The model under review builds one solid part; all positions refer to its coordinate system, in mm. A direction names the side the tool comes from. Coordinates: 2 decimals unless noted, no trailing zeros. Order: outer loops, then holes, each group sorted by start corner. A loop starts at its lowest first (then second) coordinate and runs counter-clockwise, first axis right, second up.
```python
from build123d import *

# Parameters (mm, degrees)
EXTRUDE_1_DEPTH                  = 10.5
SKETCH_2_W                       = 102.00000000000001
SKETCH_2_H                       = 75.00000000000009
EXTRUDE_2_DEPTH                  = 19.4993693487819
EXTRUDE_3_DEPTH                  = 18.000000000000004
SKETCH_4_W                       = 18.000000000000004
SKETCH_4_H                       = 140
EXTRUDE_4_DEPTH                  = 70.0006306512181
EXTRUDE_START                    = 10.499999999999998
EXTRUDE_5_DEPTH                  = 10.499999999999998
CUT_EXTRUDE_1_REACH              = 194.401
SKETCH_7_W                       = 4.000000000000014
SKETCH_7_H                       = 29.999999999999993
CUT_EXTRUDE_2_DEPTH              = 201.0099997500125
CUT_EXTRUDE_3_DEPTH              = 210.76176963403032
CUT_EXTRUDE_4_DEPTH              = 210.76176963403032
EXTRUDE_6_DEPTH                  = 0.7500000000000007
HOLE_WIZARD_M521_D               = 61.5
EXTRUDE_7_DEPTH                  = 5.749999999999998
HOLE_WIZARD_6_7_6_7_1_AT_2_COUNT = 2
HOLE_WIZARD_6_7_6_7_1_AT_2_PITCH = 45
HOLE_WIZARD_4_0_4_1_AT_2_COUNT   = 2
HOLE_WIZARD_4_0_4_1_AT_2_PITCH   = 49.49747468305833
CHAMFER_1_SIZE                   = 0.9999999999999991
EXTRUDE_START_2                  = -16.249369
SKETCH_28_R                      = 3.35
SKETCH_28_R_2                    = 9.999999999999993
SKETCH_28_R_3                    = 3.350000000000003
EXTRUDE_8_DEPTH                  = 16.249369
SKETCH_30_R                      = 3.0000000000000018
CUT_EXTRUDE_5_DEPTH              = 7
EXTRUDE_START_3                  = -21.000000000000007
SKETCH_32_R                      = 2.9999999999999933
EXTRUDE_9_DEPTH                  = 21.000000000000007


with BuildPart() as part:
    # Эскиз1 → Бобышка-Вытянуть1 (new body)
    with BuildSketch(Plane(origin=(29.9993693487819, 0, 0), x_dir=(0, 0, -1), z_dir=(1, 0, 0))):
        with BuildLine():
            Line((14.919229074297327, 90.0005475751909), (0, 90.0005475751909))
            Line((0, 90.0005475751909), (0, 15.0005475751908))
            Line((0, 15.0005475751908), (102.00000000000001, 15.0005475751908))
            Line((102.00000000000001, 15.0005475751908), (85.69382268537409, 20.93551075238141))
            ThreePointArc((85.69382268537409, 20.93551075238141), (74.94644857866616, 27.70982740688085), (67.9664449575318, 38.324768093192546))
            ThreePointArc((67.9664449575318, 38.324768093192546), (24.088528585175357, 46.3477790832992), (14.919229074297327, 90.0005475751909))
        make_face()
    extrude(amount=-EXTRUDE_1_DEPTH)

    # Эскиз2 → Бобышка-Вытянуть2 (add)
    with BuildSketch(Plane.ZY.offset(-19.4993693487819)):
        with Locations((-51.00000000000001, 52.50054757519085)):
            Rectangle(SKETCH_2_W, SKETCH_2_H)
    extrude(amount=EXTRUDE_2_DEPTH)

    # Эскиз3 → Бобышка-Вытянуть3 (add)
    with BuildSketch(Plane.XY):
        Polygon((29.999369348781915, -6.94e-15), (3.47e-15, 15.000547575190799), (0, 124.997494914823), (29.997641385548, 140), (29.999369348781904, 140), align=None)
    extrude(amount=EXTRUDE_3_DEPTH)

    # Эскиз4 → Бобышка-Вытянуть4 (add)
    with BuildSketch(Plane(origin=(29.9993693487819, 0, 0), x_dir=(0, 0, -1), z_dir=(1, 0, 0))):
        with Locations((-9.000000000000002, 70)):
            Rectangle(SKETCH_4_W, SKETCH_4_H)
    extrude(amount=EXTRUDE_4_DEPTH)

    # Эскиз5 → Бобышка-Вытянуть5 (add)
    with BuildSketch(Plane(origin=(19.4993693487819, 0, 0), x_dir=(0, 0, -1), z_dir=(1, 0, 0)).offset(EXTRUDE_START)):
        with BuildLine():
            Line((89.08077092570272, 90.0005475751909), (102.00000000000001, 90.0005475751909))
            Line((102.00000000000001, 90.0005475751909), (102.00000000000001, 23.000547575190808))
            Line((102.00000000000001, 23.000547575190808), (91.92678266011816, 26.666898850201964))
            ThreePointArc((91.92678266011816, 26.666898850201964), (81.8910585435448, 32.765618882150974), (74.9654117449494, 42.24958224106233))
            ThreePointArc((74.9654117449494, 42.24958224106233), (90.35915387380979, 63.660894475956894), (89.08077092570272, 90.0005475751909))
        make_face()
    extrude(amount=-EXTRUDE_5_DEPTH)

    # Эскиз6 → Вырез-Вытянуть1 (cut, up to next)
    with BuildSketch(Plane(origin=(16.2493693487819, 0, 0), x_dir=(0, -1, 0), z_dir=(-1, 0, 0)), mode=Mode.PRIVATE) as cut_extrude_1_sk1:
        with BuildLine():
            Line((-90.0005475751909, -14.919229074297327), (-90.0005475751909, -89.08077092570272))
            ThreePointArc((-90.0005475751909, -89.08077092570272), (-34.999999999999936, -52), (-90.0005475751909, -14.919229074297327))
        make_face()
    cut_extrude_1_tool1 = extrude(cut_extrude_1_sk1.sketch, amount=-CUT_EXTRUDE_1_REACH, mode=Mode.PRIVATE) & part.part
    add(cut_extrude_1_tool1.solids().sort_by_distance((16.249369, 65.774947, -52))[0], mode=Mode.SUBTRACT)

    # Эскиз7 → Вырез-Вытянуть2 (cut, through all)
    with BuildSketch(Plane.ZY):
        with Locations((-100, 75.0005475751909)):
            Rectangle(SKETCH_7_W, SKETCH_7_H)
    extrude(amount=-CUT_EXTRUDE_2_DEPTH, mode=Mode.SUBTRACT)

    # Эскиз8 → Вырез-Вытянуть3 (cut, through all)
    with BuildSketch(Plane.XY.offset(18.000000000000004)):
        with BuildLine():
            Line((64, 140), (45.999999999999986, 140))
            Line((45.999999999999986, 140), (46, 120))
            ThreePointArc((46, 120), (55, 111), (64, 120))
            Line((64, 120), (64, 140))
        make_face()
    extrude(amount=-CUT_EXTRUDE_3_DEPTH, mode=Mode.SUBTRACT)

    # Эскиз9 → Вырез-Вытянуть4 (cut, through all)
    with BuildSketch(Plane.XY.offset(18.000000000000004)):
        with BuildLine():
            Line((46.00000000000001, 0), (64, 0))
            Line((64, 0), (64, 20.000000000000004))
            ThreePointArc((64, 20.000000000000004), (55, 29), (45.999999999999986, 20.000000000000004))
            Line((45.999999999999986, 20.000000000000004), (46.00000000000001, 0))
        make_face()
    extrude(amount=-CUT_EXTRUDE_4_DEPTH, mode=Mode.SUBTRACT)

    # Эскиз10 → Бобышка-Вытянуть6 (add)
    with BuildSketch(Plane(origin=(16.2493693487819, 0, 0), x_dir=(0, 0, -1), z_dir=(1, 0, 0))):
        with BuildLine():
            Line((15.729542704227807, 90.0005475751909), (88.27045729577222, 90.00054757519085))
            ThreePointArc((88.27045729577222, 90.00054757519085), (51.999999999999986, 35.75000000000001), (15.729542704227807, 90.0005475751909))
        make_face()
    extrude(amount=EXTRUDE_6_DEPTH)

    # Отверстие с зазором M521 (through all)
    with Locations(Plane(origin=(16.999369348781904, 0, 0), x_dir=(0, 0, -1), z_dir=(1, 0, 0))):
        with Locations((52, 75)):
            Hole(HOLE_WIZARD_M521_D / 2)

    # Эскиз20 → Диаметр отверстия Ø4.0 (4)1 (revolve, cut)
    with BuildSketch(Plane(origin=(16.999369348781904, 75, -17), x_dir=(0, 0, -1), z_dir=(0, 1, 0))):
        Polygon((0, 0), (-4.16e-15, 16.999369348781904), (1.9999999999999978, 16.999369348781904), (1.9999999999999896, -1.31e-15), align=None)
    hole_wizard_4_0_4_1 = revolve(axis=Axis((23.349369348781895, 75, -17), (-1, 0, 0)), mode=Mode.SUBTRACT)

    # Диаметр отверстия Ø4.0 (4)1 at 2: Диаметр отверстия Ø4.0 (4)1 ×2
    with Locations(*[Vector(0, -0.7071067811865475, -0.7071067811865477) * (i * HOLE_WIZARD_4_0_4_1_AT_2_PITCH) for i in range(1, HOLE_WIZARD_4_0_4_1_AT_2_COUNT)]):
        add(hole_wizard_4_0_4_1, mode=Mode.SUBTRACT)

    # Эскиз22 → Диаметр отверстия Ø6.0 (6)1 (revolve, cut)
    with BuildSketch(Plane(origin=(29.9993693487819, 40.0005475751908, -90), x_dir=(0, 0, -1), z_dir=(0, 1, 0))):
        Polygon((0, 0), (-7.35e-15, 30.000369348781906), (2.9999999999999867, 30.000369348781906), (2.9999999999999907, -1.19e-15), align=None)
    revolve(axis=Axis((36.34936934878189, 40.0005475751908, -90), (-1, 0, 0)), mode=Mode.SUBTRACT)


with BuildPart() as body_2:
    # Эскиз13 → Бобышка-Вытянуть7 (new body)
    with BuildSketch(Plane(origin=(16.2493693487819, 0, 0), x_dir=(0, -1, 0), z_dir=(-1, 0, 0))):
        with BuildLine():
            Line((-90.0005475751909, -26.01955403684463), (-90.0005475751909, -77.98044596315543))
            ThreePointArc((-90.0005475751909, -77.98044596315543), (-44.99999999999993, -51.99999999999999), (-90.0005475751909, -26.01955403684463))
        make_face()
    extrude(amount=-EXTRUDE_7_DEPTH)

    # Эскиз16 → Диаметр отверстия Ø6.7 (6.7)1 (revolve, cut)
    with BuildSketch(Plane(origin=(21.9993693487819, 75, -74.5), x_dir=(0, 0, -1), z_dir=(0, 1, 0))):
        Polygon((0, 0), (-1.41e-15, 5.7509999999999994), (3.3500000000000045, 5.7509999999999994), (3.3499999999999934, -1.15e-15), align=None)
    hole_wizard_6_7_6_7_1 = revolve(axis=Axis((28.34936934878189, 75, -74.5), (-1, 0, 0)), mode=Mode.SUBTRACT)

    # Диаметр отверстия Ø6.7 (6.7)1 at 2: Диаметр отверстия Ø6.7 (6.7)1 ×2
    with Locations(*[(0, 0, i * HOLE_WIZARD_6_7_6_7_1_AT_2_PITCH) for i in range(1, HOLE_WIZARD_6_7_6_7_1_AT_2_COUNT)]):
        add(hole_wizard_6_7_6_7_1, mode=Mode.SUBTRACT)

    # Эскиз18 → Диаметр отверстия Ø20.0 (20)1 (revolve, cut)
    with BuildSketch(Plane(origin=(21.9993693487819, 75, -52.00000000000001), x_dir=(0, 0, -1), z_dir=(0, 1, 0))):
        Polygon((0, 0), (-1.41e-15, 5.7510000000000066), (9.99999999999999, 5.7510000000000066), (9.99999999999999, -3.3e-16), align=None)
    revolve(axis=Axis((28.34936934878189, 75, -52.00000000000001), (-1, 0, 0)), mode=Mode.SUBTRACT)


with BuildPart() as hole_wizard_5_0_5_1_tool:
    # Эскиз24 → Диаметр отверстия Ø5.0 (5)1 (revolve)
    with BuildSketch(Plane(origin=(23, 75.0005475751909, -98), x_dir=(0, 1, 0), z_dir=(1, 0, 0))):
        Polygon((0, 0), (-1.127e-14, 45.999999999999986), (2.499999999999981, 45.999999999999986), (2.4999999999999867, -1.25e-15), align=None)
    revolve(axis=Axis((23, 75.0005475751909, -104.35), (0, 0, 1)))


with BuildPart() as part_1:
    add(part.part)

    # Диаметр отверстия Ø5.0 (5)1: cut by hole_wizard_5_0_5_1_tool
    add(hole_wizard_5_0_5_1_tool.part, mode=Mode.SUBTRACT)

    # Эскиз26 → Отверстие с зазором M61 (revolve, cut)
    with BuildSketch(Plane(origin=(15.8866729980809, 33.128633292951, -102.00000000000001), x_dir=(0, 1, 0), z_dir=(1, 0, 0))):
        Polygon((0, 0), (-1.47e-15, 5.999999999999993), (3.2357711959407984, 6.000000000000005), (3.2357711959408, -1.16e-15), align=None)
    revolve(axis=Axis((15.8866729980809, 33.128633292951, -108.35000000000001), (0, 0, 1)), mode=Mode.SUBTRACT)


with BuildPart() as body_2_1:
    add(body_2.part)

    # Диаметр отверстия Ø5.0 (5)1: cut by hole_wizard_5_0_5_1_tool
    add(hole_wizard_5_0_5_1_tool.part, mode=Mode.SUBTRACT)

    # Фаска1
    chamfer_1_edges = [body_2_1.edges().sort_by_distance(p)[0] for p in [
        (21.9993693487819, 74.99943746278025, -42.00000001582242),
    ]]
    chamfer(chamfer_1_edges, length=CHAMFER_1_SIZE)


with BuildPart() as extrude_8_tool:
    # Эскиз28 → Бобышка-Вытянуть8 (new body)
    with BuildSketch(Plane.ZY.offset(EXTRUDE_START_2)):
        with BuildLine():
            Line((-78.84298926059529, 90.0005475751909), (-25.157010739404722, 90.0005475751909))
            ThreePointArc((-25.157010739404722, 90.0005475751909), (-52.000000000000014, 44.250000000000014), (-78.84298926059529, 90.0005475751909))
        make_face()
        with Locations(Location((-29.500000000000004, 75, 0), (0, 0, 180))):
            Circle(SKETCH_28_R, mode=Mode.SUBTRACT)
        with Locations(Location((-52.00000000000001, 75, 0), (0, 0, 188.618876561))):
            Circle(SKETCH_28_R_2, mode=Mode.SUBTRACT)
        with Locations(Location((-74.5, 75, 0), (0, 0, 223.135094042))):
            Circle(SKETCH_28_R_3, mode=Mode.SUBTRACT)
    extrude(amount=EXTRUDE_8_DEPTH)


with BuildPart() as part_2:
    add(part_1.part)


with BuildPart() as part_3:
    # Бобышка-Вытянуть8: joined with extrude_8_tool
    add(part_2.part.fuse(extrude_8_tool.part, body_2_1.part, tol=0.00001))

    # Эскиз30 → Вырез-Вытянуть5 (cut)
    with BuildSketch(Plane.XZ.offset(-15.0005475751908)):
        with Locations(Location((19.9993693487819, -77.00000000000001, 0), (0, 0, 270))):
            Circle(SKETCH_30_R)
    extrude(amount=-CUT_EXTRUDE_5_DEPTH, mode=Mode.SUBTRACT)

    # Эскиз32 → Бобышка-Вытянуть9 (add)
    with BuildSketch(Plane.ZY.offset(EXTRUDE_START_3)):
        with Locations(Location((-90, 40.0005475751908, 0), (0, 0, 180))):
            Circle(SKETCH_32_R)
    extrude(amount=EXTRUDE_9_DEPTH)


solid = part_3.part
```
(1) We need section D-D, the plane z = -5.5. Write out the cut boundary in (x, y), and give its area (3 significant figures).
A:
outline: (0, 15) - (30, 15) - (30, 90) - (0, 90) - close
area: 2,250 mm2
(2) We need section A-A, the plane z = -52. Write out the cut boundary in (x, y), and give its area (3 significant figures).
A:
outline: (0, 15) - (30, 15) - (30, 35) - (16.25, 35) - (16.25, 35.75) - (17, 35.75) - (17, 38) - (0, 38) - close; (0, 42) - (17, 42) - (17, 44.25) - (16.25, 44.25) - (16.25, 45) - (22, 45) - (22, 64) - (21, 65) - (0, 65) - close; (0, 85) - (21, 85) - (22, 86) - (22, 90) - (0, 90) - close
area: 1,250 mm2
(3) We need section B-B, the plane y = 10.5. Write out the cut boundary in (x, z), and give its area (3 significant figures).
A:
outline: (9, 0) - (46, 0) - (46, 18) - (9, 18) - close; (64, 0) - (100, 0) - (100, 18) - (64, 18) - close
area: 1,310 mm2
(4) We need section C-C, the plane x = 81.5. Write out the cut boundary in (y, z).
A:
outline: (0, 0) - (140, 0) - (140, 18) - (0, 18) - close
(5) Wall thickness on probe 1 along Z at (x, y) = (16, 75); probe 2 along Z at (x, y) = (9, 40); probe 3 along Z at (x, y) = (47, 27.5): over which ranges is each line inside the solid? List them lowest first.
A:
probe 1: z = -98 to -77.85, -71.15 to -62, -42 to -32.85, -26.15 to -19, -15 to 18
probe 2: z = -102 to -54, -50 to 18
probe 3: z = 0 to 18
(6) For pin 1 Ø23 at (y, z) = (75, -52) entering from +X; pin 2 Ø8 at (y, z) = (29, -13) entering from +X; pin 3 Ø3 at (x, y) = (16, 33) entering from -Z, all flat-tipped, find the tip position at first contact; note any pin that passes through.
A:
pin 1: stops at x = 22
pin 2: stops at x = 30
pin 3: stops at z = -96
(7) Draft analysis for pull direction Y (two halves, no side actions). For faces 1 (the face through (14.8, 132.4, 8.9)), 2 (the face through (11.15, 76.51, -77.49)), 3 (the face through (22.249, 77.385, -95.003)), 4 (the face through (100, 71, 9)), state which applies: released by +Y, released by -Y, zero draft, split by the parting line, or undercut.
A:
face 1: released by +Y
face 2: undercut
face 3: undercut
face 4: zero draft
(8) Machinability: for faces 5 (the face through (21.999, 63, -52)), 6 (the face through (19.499, 29, -85)), 7 (the face through (20.5, 75, -79.5)), 8 (the face through (15.7, 29.9, -99)), which of the approach directions +Z, -Z, +X, -X, +Y, -Y give a long, thin tool a straight path to every point of the face, cutting with its end or side? Answer none if there is none.
A:
face 5: +X, +Y
face 6: +X
face 7: -Z, +X
face 8: -Z
